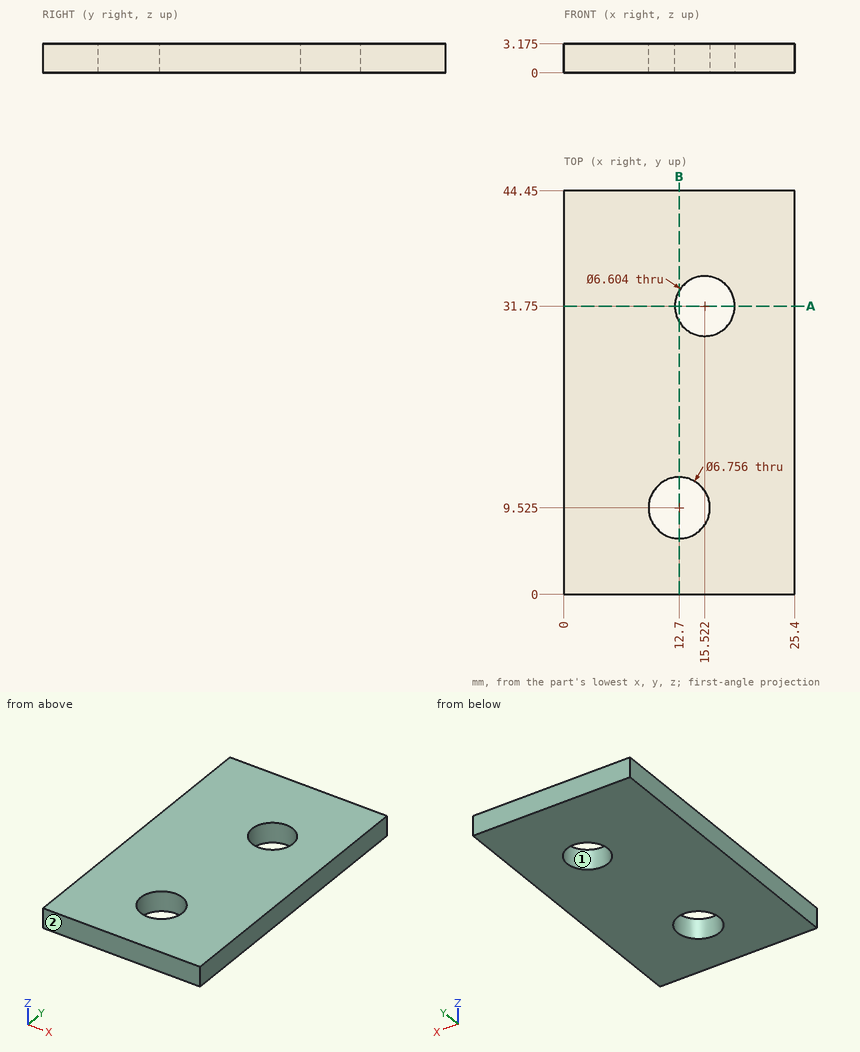
Check sheet for the drawn part. Datum: minimum x, y, z corner. Units: mm. Round coordinates to 2 decimals unless told otherwise and drop trailing zeros. Loops run counter-clockwise (first coordinate to the right, second up) from the corner with the lowest first, then second, coordinate; pieces in that order, holes last. Notation, with made-up numbers: (81, -8.5) - (136, -8.5) arc R33 cw to (136, 25.5) - close; hole circle Ø7 at (87.25, 15). An arc over 180 degrees is marked (long way). Write each question's results on one line, items separated by ' | '. Start each with the question number.
Q1. Gauge pin test, flat end, axial feed: P1, Ø6, axis at x = 21, y = 16.5, coming from the -Z side. Record the tip position at first contact, or that the pin passes through.
Q2. Release check for a two-part mould opening along X. For the marked faces 1 and 2 record: +X half, -X half, draft (parallel to the pull), parting line (faces both ways), or undercut.
Q3. Thickness scan on line 1 (X direction, y = 31.5, z = 2.85) (1 decimal); line 2 (X direction, y = 31, z = 1.8). Record the ranges inside material, lowest first. Write a range as [from, to].
Q4. Cross-section at A-A on y = 31.75. Enter the section's corners in (x, z) (1 decimal).
Q5. Cross-section at B-B on x = 12.7. State how many separate pieces and enclosed holes the cut face has, and give its area (3 significant figures).
Answers below:
1) P1: stops at z = 0
2) face 1: undercut | face 2: draft
3) line 1: x = [0, 12.2], [18.8, 25.4] | line 2: x = [0, 12.31], [18.74, 25.4]
4) outline: (0, 0) - (12.2, 0) - (12.2, 3.2) - (0, 3.2) - close; (18.8, 0) - (25.4, 0) - (25.4, 3.2) - (18.8, 3.2) - close
5) separate pieces: 3 | enclosed holes: 0 | area: 109 mm²
